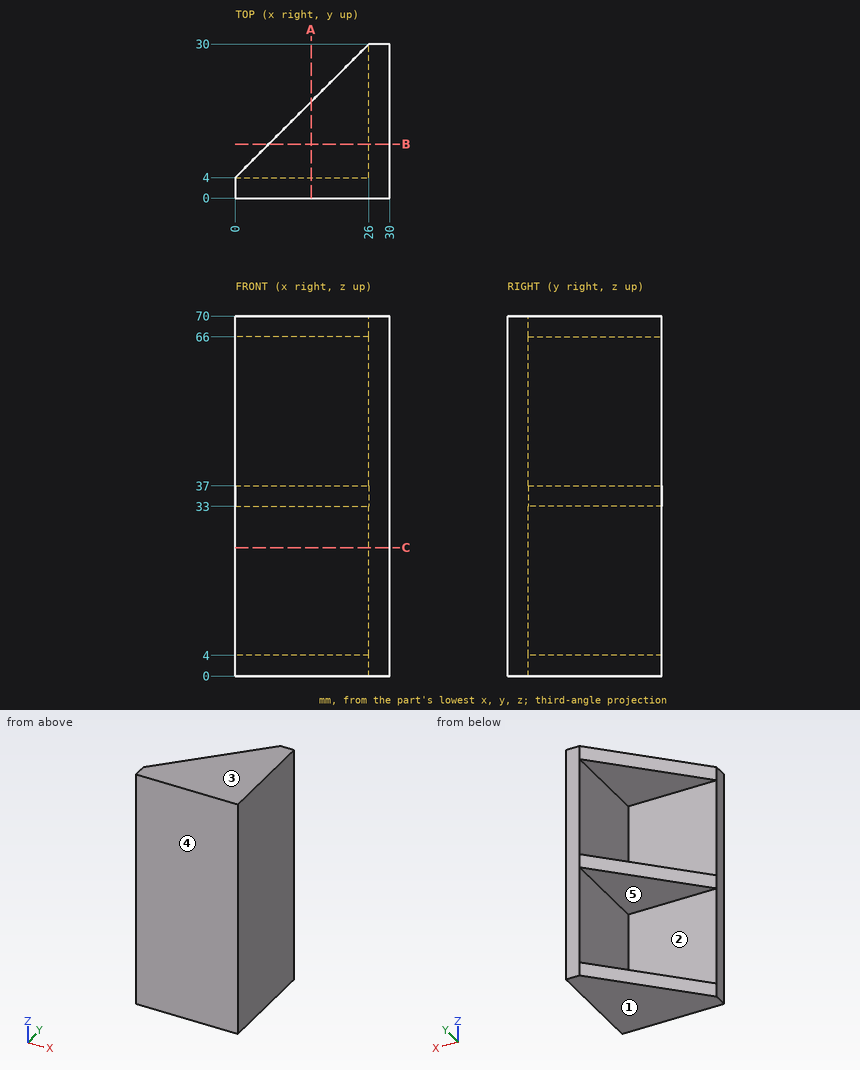
The figure shows three views and two pictorial views of one solid part (mm, origin at its lowest corner). Answer the questions. A direction names the side the tool comes from. Give positions to 0.01 mm unless a question says otherwise; leave off trailing zeros. Order: outer loops, then holes, each group sorted by start corner. A loop starts at its lowest first (then second) coordinate and runs counter-clockwise, first axis right, second up. Notation, with made-up numbers: (47, 56.5) -> (105, 56.5) arc R22 ccw to (105, 63.5) -> close; hole circle Ø11 at (22, -15.5). An arc over 180 degrees is marked (long way). One line per item, written item: value.
1) Determine the mould class of the marked faces 3, 4 and 5 for opening direction Z: pulls with the +Z half, pulls with the -Z half, needs draft (parallel to the pull), parting line crosses it, or undercut.
Reported:
face 3: pulls with the +Z half
face 4: needs draft
face 5: undercut
2) A tool of negligible diameter and unlimited length cuts with its end or side. For the marked faces 1 and 2, from which of +Z, -Z, +X, -X, +Y, -Y can it reach the whole face along a straight path? Write none if from no direction.
Reported:
face 1: -Z, +X, -X, +Y, -Y
face 2: -X, +Y
3) Flat-ended cylindrical pins translate along their axes: P1, Ø1, axis at y = 7.5, z = 29, coming from the -X side; P2, Ø1.5, axis at x = 24, z = 35.5, coming from the +Y side; P3, Ø13, axis at x = 14.5, z = 46.5, coming from the +Y side. Find the tip coordinate at first contact, or state that the pin passes through.
Reported:
P1: stops at x = 26
P2: stops at y = 28.75
P3: stops at y = 4
4) Find section C-C, the plane z = 25. Determine the outline of the cut face in (x, y).
Reported:
outline: (0, 0) -> (30, 0) -> (30, 30) -> (26, 30) -> (26, 4) -> (0, 4) -> close
5) Find section A-A, the plane x = 14.75. Determine the outline of the cut face in (y, z), plus the area to 3 significant figures.
Reported:
outline: (0, 0) -> (18.75, 0) -> (18.75, 4) -> (4, 4) -> (4, 33) -> (18.75, 33) -> (18.75, 37) -> (4, 37) -> (4, 66) -> (18.75, 66) -> (18.75, 70) -> (0, 70) -> close
area: 457 mm^2
6) Find the intervals of material crossed by line 1 (Z direction, x = 19.25, y = 18.25); line 2 (Y direction, x = 8.5, z = 47.5); line 3 (X direction, y = 12, z = 65.5), in increasing order.
Reported:
line 1: z = 0 to 4, 33 to 37, 66 to 70
line 2: y = 0 to 4
line 3: x = 26 to 30
7) Find section B-B, the plane y = 10.5. Determine the outline of the cut face in (x, z).
Reported:
outline: (6.5, 0) -> (30, 0) -> (30, 70) -> (6.5, 70) -> (6.5, 66) -> (26, 66) -> (26, 37) -> (6.5, 37) -> (6.5, 33) -> (26, 33) -> (26, 4) -> (6.5, 4) -> close
